```python
from build123d import *

# Parameters (mm, degrees)
SKETCH1_W           = 185
SKETCH1_H           = 84
SKETCH1_R           = 2.25
BOSS_EXTRUDE1_DEPTH = 5
SKETCH2_W           = 185
SKETCH2_H           = 79
SKETCH2_R           = 2.25
BOSS_EXTRUDE2_DEPTH = 3
CHAMFER1_SIZE       = 8
CHAMFER3_SIZE       = 3
SKETCH3_W           = 7.071067812
SKETCH3_H           = 2.6
CUT_EXTRUDE1_DEPTH  = 221.270985121
SKETCH4_W           = 115.2
SKETCH4_H           = 34.6
CUT_EXTRUDE2_DEPTH  = 204.334699449


with BuildPart() as part:
    # Sketch1 → Boss-Extrude1 (new body)
    with BuildSketch(Plane.XY):
        with Locations((92.5, 42)):
            Rectangle(SKETCH1_W, SKETCH1_H)
        with Locations((15, 9)):
            Circle(SKETCH1_R, mode=Mode.SUBTRACT)
        with Locations(Location((170, 9, 0), (0, 0, 180))):
            Circle(SKETCH1_R, mode=Mode.SUBTRACT)
        with Locations((15, 72)):
            Circle(SKETCH1_R, mode=Mode.SUBTRACT)
        with Locations(Location((170, 72, 0), (0, 0, 180))):
            Circle(SKETCH1_R, mode=Mode.SUBTRACT)
    extrude(amount=-BOSS_EXTRUDE1_DEPTH)

    # Sketch2 → Boss-Extrude2 (add)
    with BuildSketch(Plane(origin=(0, 0, -5), x_dir=(-1, 0, 0), z_dir=(0, 0, -1))):
        with Locations((-92.5, 44.5)):
            Rectangle(SKETCH2_W, SKETCH2_H)
        with Locations(Location((-15, 9, 0), (0, 0, 180))):
            Circle(SKETCH2_R, mode=Mode.SUBTRACT)
        with Locations((-170, 9)):
            Circle(SKETCH2_R, mode=Mode.SUBTRACT)
        with Locations(Location((-15, 72, 0), (0, 0, 180))):
            Circle(SKETCH2_R, mode=Mode.SUBTRACT)
        with Locations((-170, 72)):
            Circle(SKETCH2_R, mode=Mode.SUBTRACT)
    extrude(amount=BOSS_EXTRUDE2_DEPTH)

    # Chamfer1
    # the kernel refuses this chamfer: 8 mm, written as the material it takes off along each edge
    with BuildSketch(Plane(origin=(185, -15.573463904, -8), x_dir=(-0.9996219169112968, 0, -0.027495876610586296), z_dir=(0, 1, 0)), Plane(origin=(0, 104.573463904, -8), x_dir=(0.9996219169112968, 0, -0.027495876610586275), z_dir=(0, -1, 0))) as chamfer1_piece_1:
        Polygon((CHAMFER1_SIZE * 0.999621916911, CHAMFER1_SIZE * 0.0274958766106), (-CHAMFER1_SIZE * 0.0274958766106, CHAMFER1_SIZE * 0.999621916911), (0, 0), align=None)
    extrude(amount=120.146927807, mode=Mode.SUBTRACT)

    # Chamfer3
    chamfer3_edges = [part.edges().sort_by_distance(p)[0] for p in [
        (92.5, 84, -8),
    ]]
    chamfer(chamfer3_edges, length=CHAMFER3_SIZE)

    # Sketch3 → Cut-Extrude1 (cut, through all, along a direction that is not the sketch's normal)
    with BuildSketch(Plane(origin=(92.5, 0, -92.5), x_dir=(-0.7071067811865452, 0, -0.7071067811865498), z_dir=(0.7071067811865498, 0, -0.7071067811865452))):
        with Locations((-127.279220614, 1.3)):
            Rectangle(SKETCH3_W, SKETCH3_H)
    extrude(amount=-CUT_EXTRUDE1_DEPTH, dir=(1, 0, 0), mode=Mode.SUBTRACT)

    # Sketch4 → Cut-Extrude2 (cut, through all)
    with BuildSketch(Plane.XY):
        with Locations((92.5, 19.9)):
            Rectangle(SKETCH4_W, SKETCH4_H)
        with BuildLine():
            Line((37.4, 76), (37.4, 56))
            ThreePointArc((37.4, 56), (34.9, 53.5), (32.4, 56))
            Line((32.4, 56), (32.4, 76))
            ThreePointArc((32.4, 76), (34.9, 78.5), (37.4, 76))
        make_face()
        with BuildLine():
            Line((47, 76), (47, 56))
            ThreePointArc((47, 56), (44.5, 53.5), (42, 56))
            Line((42, 56), (42, 76))
            ThreePointArc((42, 76), (44.5, 78.5), (47, 76))
        make_face()
        with BuildLine():
            Line((56.6, 76), (56.6, 56))
            ThreePointArc((56.6, 56), (54.1, 53.5), (51.6, 56))
            Line((51.6, 56), (51.6, 76))
            ThreePointArc((51.6, 76), (54.1, 78.5), (56.6, 76))
        make_face()
        with BuildLine():
            Line((66.2, 76), (66.2, 56))
            ThreePointArc((66.2, 56), (63.7, 53.5), (61.2, 56))
            Line((61.2, 56), (61.2, 76))
            ThreePointArc((61.2, 76), (63.7, 78.5), (66.2, 76))
        make_face()
        with BuildLine():
            Line((75.8, 76), (75.8, 56))
            ThreePointArc((75.8, 56), (73.3, 53.5), (70.8, 56))
            Line((70.8, 56), (70.8, 76))
            ThreePointArc((70.8, 76), (73.3, 78.5), (75.8, 76))
        make_face()
        with BuildLine():
            Line((85.4, 76), (85.4, 56))
            ThreePointArc((85.4, 56), (82.9, 53.5), (80.4, 56))
            Line((80.4, 56), (80.4, 76))
            ThreePointArc((80.4, 76), (82.9, 78.5), (85.4, 76))
        make_face()
        with BuildLine():
            Line((95, 76), (95, 56))
            ThreePointArc((95, 56), (92.5, 53.5), (90, 56))
            Line((90, 56), (90, 76))
            ThreePointArc((90, 76), (92.5, 78.5), (95, 76))
        make_face()
        with BuildLine():
            Line((104.6, 76), (104.6, 56))
            ThreePointArc((104.6, 56), (102.1, 53.5), (99.6, 56))
            Line((99.6, 56), (99.6, 76))
            ThreePointArc((99.6, 76), (102.1, 78.5), (104.6, 76))
        make_face()
        with BuildLine():
            Line((114.2, 76), (114.2, 56))
            ThreePointArc((114.2, 56), (111.7, 53.5), (109.2, 56))
            Line((109.2, 56), (109.2, 76))
            ThreePointArc((109.2, 76), (111.7, 78.5), (114.2, 76))
        make_face()
        with BuildLine():
            Line((123.8, 76), (123.8, 56))
            ThreePointArc((123.8, 56), (121.3, 53.5), (118.8, 56))
            Line((118.8, 56), (118.8, 76))
            ThreePointArc((118.8, 76), (121.3, 78.5), (123.8, 76))
        make_face()
        with BuildLine():
            Line((133.4, 76), (133.4, 56))
            ThreePointArc((133.4, 56), (130.9, 53.5), (128.4, 56))
            Line((128.4, 56), (128.4, 76))
            ThreePointArc((128.4, 76), (130.9, 78.5), (133.4, 76))
        make_face()
        with BuildLine():
            Line((143, 76), (143, 56))
            ThreePointArc((143, 56), (140.5, 53.5), (138, 56))
            Line((138, 56), (138, 76))
            ThreePointArc((138, 76), (140.5, 78.5), (143, 76))
        make_face()
        with BuildLine():
            Line((152.6, 76), (152.6, 56))
            ThreePointArc((152.6, 56), (150.1, 53.5), (147.6, 56))
            Line((147.6, 56), (147.6, 76))
            ThreePointArc((147.6, 76), (150.1, 78.5), (152.6, 76))
        make_face()
    extrude(amount=-CUT_EXTRUDE2_DEPTH, mode=Mode.SUBTRACT)


solid = part.part
```
Could you check a few things on this model? Use its own coordinates, in mm. A direction names the side the tool comes from. Round coordinates to 2 decimals unless told otherwise and drop trailing zeros. Write each loop counter-clockwise with the first axis right and the second up, starting at its lowest first coordinate (ties: lowest second). Pieces come first, ordered by that corner, then holes.
(1) Suppose I cut it at A-A on x = 140.5. Write out the boundary of the cut face in (y, z), and give its area (3 significant figures).
Findings below:
outline: (37.2, -8) - (53.5, -8) - (53.5, 0) - (37.2, 0) - close; (78.5, -8) - (81, -8) - (84, -5) - (84, 0) - (78.5, 0) - close
area: 170 mm2
(2) Which directions (+Z, -Z, +X, -X, +Y, -Y) give clear straight access to the entire face, cutting with the end or side of a thin tool? Please do faces 1 (the face through (92.6, 53.5, -3.9)), 2 (the face through (19, 2.6, -3)).
Findings below:
face 1: +Z, -Z
face 2: +Z, -Z, +X, -X, -Y
(3) For pin 1 (3 mm diameter, centred on x = 88.5, z = -7, fed in from +Y); pin 2 (4 mm diameter, centred on y = 73, z = -7, fed in from +X); pin 3 (2.5 mm diameter, centred on y = 68, z = -2.5, fed in from -X), each with a flat end and sliding along its axis, tell me the tip position at first contact or that it passes through.
Findings below:
pin 1: stops at y = 83.5
pin 2: stops at x = 180
pin 3: stops at x = 1.25
(4) If I drill on probe 1 along Y at (x, z) = (170, -3.2); probe 2 along Y at (x, z) = (170, -5.95); probe 3 along Y at (x, z) = (60.5, -0.25), over which ranges is the centre line in solid material (lowest first)?
Findings below:
probe 1: y = 2.6 to 6.75, 11.25 to 69.75, 74.25 to 84
probe 2: y = 5 to 6.75, 11.25 to 69.75, 74.25 to 83.05
probe 3: y = 37.2 to 84
(5) Suppose I cut it at D-D on y = 72. State how many separate pieces and enclosed holes the cut face has, and give its area (3 significant figures).
Findings below:
separate pieces: 16
enclosed holes: 0
area: 824 mm2
(6) Suppose I cut it at C-C on x = 170. Write out the boundary of the cut face in (y, z), and give its area (4 significant figures).
Findings below:
outline: (2.6, -5) - (5, -5) - (5, -8) - (6.75, -8) - (6.75, 0) - (2.6, 0) - close; (11.25, -8) - (69.75, -8) - (69.75, 0) - (11.25, 0) - close; (74.25, -8) - (81, -8) - (84, -5) - (84, 0) - (74.25, 0) - close
area: 567.5 mm2
(7) Suppose I cut it at B-B on y = 25.5. Write out the boundary of the cut face in (x, z).
Findings below:
outline: (0, 0) - (8, -8) - (34.9, -8) - (34.9, 0) - close; (150.1, -8) - (177, -8) - (185, 0) - (150.1, 0) - close
(8) Thinking about a two-plate mould opening in X: for faces 3 (the face through (92.4, 78.5, -3.9)), 4 (the face through (4, 44, -4)), 5 (the face through (166, 2.6, -2)), 6 (the face through (181, 43, -4)), which applies, +X half, -X half, draft (parallel to the pull), parting line (faces both ways), or undercut?
Findings below:
face 3: undercut
face 4: -X half
face 5: draft
face 6: +X half
